Input: dimensioned drawing with shaded views. Units: mm. Origin: part minimum x, y, z. Coordinates: 2 decimals unless noted, no trailing zeros. Write each loop counter-clockwise with the first axis right and the second up, starting at its lowest first coordinate (ties: lowest second). Pieces come first, ordered by that corner, then holes. Notation, with made-up numbers: (77.25, -10) - (87.25, -10) arc R22 cw to (87.25, 3) - close; hole circle Ø5 at (22, 36.25). An arc over 180 degrees is marked (long way). One line per question, with ' | ' between items.
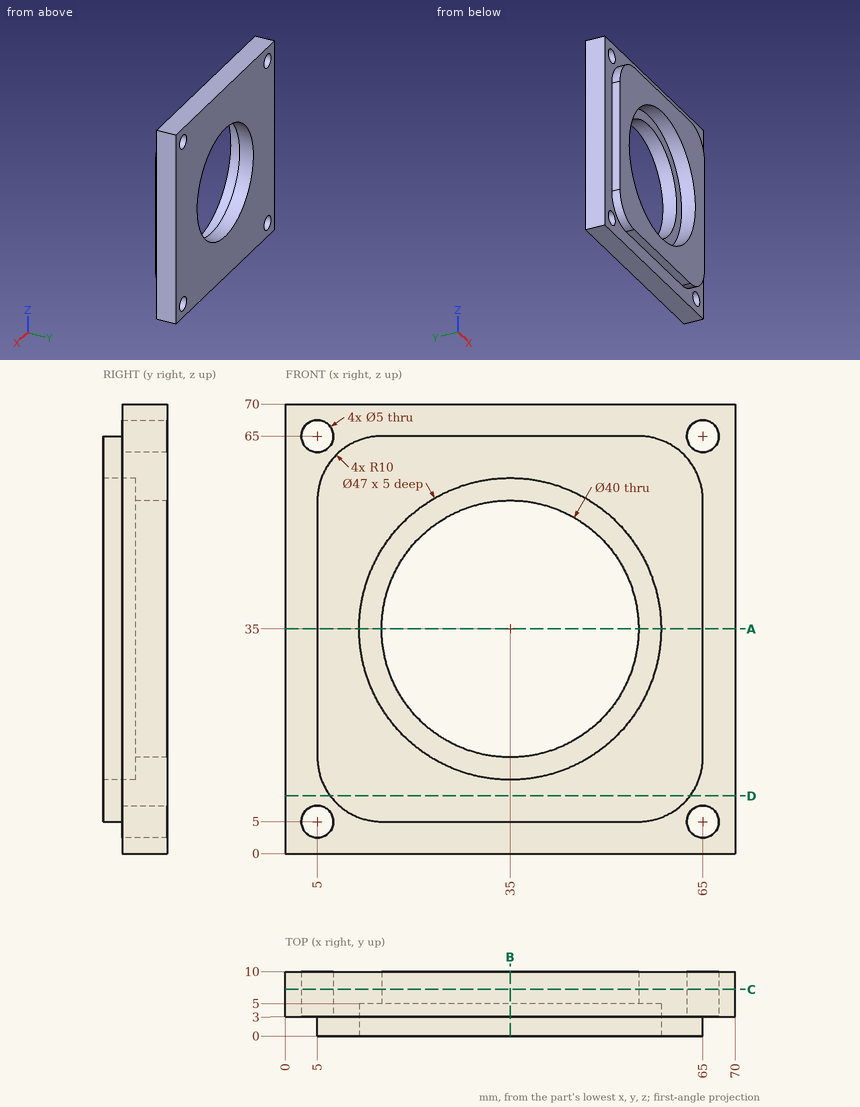
Item 1: Pin query (flat end, axial travel): pin 1 Ø3.5 at (x, y) = (40, 1) entering from +Z; pin 2 Ø1.5 at (y, z) = (4, 50.5) entering from -X; pin 3 Ø0.9 at (x, y) = (25, 2) entering from -Z; pin 4 Ø8 at (x, z) = (5, 5) entering from -Y. Return the tip coordinate at first contact, or that it passes through.
Check sheet entries:
pin 1: z = 65 | pin 2: x = 0 | pin 3: z = 5 | pin 4: y = 3
Item 2: Cut plane D-D on z = 9. Return loops of the section in (x, y).
Check sheet entries:
outline: (0, 3) - (7, 3) - (7, 0) - (63, 0) - (63, 3) - (70, 3) - (70, 10) - (0, 10) - close
Item 3: Cut plane C-C on y = 7.25. Return loops of the section in (x, z).
Check sheet entries:
outline: (0, 0) - (70, 0) - (70, 70) - (0, 70) - close; hole circle Ø5 at (5, 5); hole circle Ø5 at (5, 65); hole circle Ø40 at (35, 35); hole circle Ø5 at (65, 5); hole circle Ø5 at (65, 65)
Item 4: Cut plane B-B on x = 35. Return loops of the section in (y, z).
Check sheet entries:
outline: (0, 5) - (3, 5) - (3, 0) - (10, 0) - (10, 15) - (5, 15) - (5, 11.5) - (0, 11.5) - close; (0, 58.5) - (5, 58.5) - (5, 55) - (10, 55) - (10, 70) - (3, 70) - (3, 65) - (0, 65) - close
Item 5: Cut plane A-A on z = 35. Return loops of the section in (x, y), and give its area (3 significant figures).
Check sheet entries:
outline: (0, 3) - (5, 3) - (5, 0) - (11.5, 0) - (11.5, 5) - (15, 5) - (15, 10) - (0, 10) - close; (55, 5) - (58.5, 5) - (58.5, 0) - (65, 0) - (65, 3) - (70, 3) - (70, 10) - (55, 10) - close | area: 235 mm²
Item 6: Ray query, line 1 along Z through (x, y) = (65, 6.75); line 2 along X through (y, z) = (6.65, 35). Return the intervals inside material, ascending. Write a range as [from, to].
Check sheet entries:
line 1: [0, 2.5], [7.5, 62.5], [67.5, 70] | line 2: [0, 15], [55, 70]
